```python
from build123d import *

# Parameters (mm, degrees)
SKETCH1_W               = 58
SKETCH1_H               = 38
BOSS_EXTRUDE1_DEPTH     = 1
CUT_EXTRUDE1_DEPTH      = 35.684290392
CUT_EXTRUDE1_DEPTH_BACK = 35.684290392
SKETCH2_W               = 17
SKETCH2_H               = 14.502040096
SKETCH3_W               = 3
SKETCH3_H               = 27
BOSS_EXTRUDE2_DEPTH     = 13
SKETCH4_W               = 42
SKETCH4_H               = 2
BOSS_EXTRUDE3_DEPTH     = 13
CUT_EXTRUDE2_START      = -42
SKETCH5_W               = 10
SKETCH5_H               = 5
CUT_EXTRUDE2_DEPTH      = 3
CUT_EXTRUDE3_REACH      = 39.027
SKETCH6_R               = 1.5


with BuildPart() as part:
    # Sketch1 → Boss-Extrude1 (new, symmetric)
    with BuildSketch(Plane(origin=(0, 0, 0), x_dir=(1, 0, 0), z_dir=(0, 1, 0))):
        Rectangle(SKETCH1_W, SKETCH1_H)
    extrude(amount=BOSS_EXTRUDE1_DEPTH, both=True)

    # Sketch2 → Cut-Extrude1 (cut, two sides: drawn at the far end of the back side and taken through both)
    with BuildSketch(Plane(origin=(0, 0, 0), x_dir=(1, 0, 0), z_dir=(0, 1, 0)).offset(-CUT_EXTRUDE1_DEPTH_BACK)):
        with Locations((0, 17.251020048)):
            Rectangle(SKETCH2_W, SKETCH2_H)
    extrude(amount=CUT_EXTRUDE1_DEPTH + CUT_EXTRUDE1_DEPTH_BACK, mode=Mode.SUBTRACT)

    # Sketch3 → Boss-Extrude2 (add)
    with BuildSketch(Plane(origin=(0, 1, 0), x_dir=(1, 0, 0), z_dir=(0, 1, 0))):
        with Locations((19.5, -4.5)):
            Rectangle(SKETCH3_W, SKETCH3_H)
        with Locations((-19.5, -4.5)):
            Rectangle(SKETCH3_W, SKETCH3_H)
    extrude(amount=BOSS_EXTRUDE2_DEPTH)

    # Sketch4 → Boss-Extrude3 (add)
    with BuildSketch(Plane(origin=(0, 1, 0), x_dir=(1, 0, 0), z_dir=(0, 1, 0))):
        with Locations((0, -18)):
            Rectangle(SKETCH4_W, SKETCH4_H)
    extrude(amount=BOSS_EXTRUDE3_DEPTH)

    # Sketch5 → Cut-Extrude2 (cut)
    with BuildSketch(Plane.ZY.offset(21).offset(CUT_EXTRUDE2_START)):
        with Locations((4, 5.5)):
            Rectangle(SKETCH5_W, SKETCH5_H)
    extrude(amount=CUT_EXTRUDE2_DEPTH, mode=Mode.SUBTRACT)

    # Sketch6 → Cut-Extrude3 (cut, up to next)
    with BuildSketch(Plane(origin=(0, 1, 0), x_dir=(1, 0, 0), z_dir=(0, 1, 0)), mode=Mode.PRIVATE) as cut_extrude3_sk1:
        with Locations(Location((-26, 15, 0), (0, 0, 270))):
            Circle(SKETCH6_R)
    cut_extrude3_tool1 = extrude(cut_extrude3_sk1.sketch, amount=-CUT_EXTRUDE3_REACH, mode=Mode.PRIVATE) & part.part
    # Sketch6 → Cut-Extrude3 (cut, up to next)
    with BuildSketch(Plane(origin=(0, 1, 0), x_dir=(1, 0, 0), z_dir=(0, 1, 0)), mode=Mode.PRIVATE) as cut_extrude3_sk2:
        with Locations(Location((-26, -15, 0), (0, 0, 90))):
            Circle(SKETCH6_R)
    cut_extrude3_tool2 = extrude(cut_extrude3_sk2.sketch, amount=-CUT_EXTRUDE3_REACH, mode=Mode.PRIVATE) & part.part
    # Sketch6 → Cut-Extrude3 (cut, up to next)
    with BuildSketch(Plane(origin=(0, 1, 0), x_dir=(1, 0, 0), z_dir=(0, 1, 0)), mode=Mode.PRIVATE) as cut_extrude3_sk3:
        with Locations(Location((26, -15, 0), (0, 0, 270))):
            Circle(SKETCH6_R)
    cut_extrude3_tool3 = extrude(cut_extrude3_sk3.sketch, amount=-CUT_EXTRUDE3_REACH, mode=Mode.PRIVATE) & part.part
    # Sketch6 → Cut-Extrude3 (cut, up to next)
    with BuildSketch(Plane(origin=(0, 1, 0), x_dir=(1, 0, 0), z_dir=(0, 1, 0)), mode=Mode.PRIVATE) as cut_extrude3_sk4:
        with Locations(Location((26, 15, 0), (0, 0, 90))):
            Circle(SKETCH6_R)
    cut_extrude3_tool4 = extrude(cut_extrude3_sk4.sketch, amount=-CUT_EXTRUDE3_REACH, mode=Mode.PRIVATE) & part.part
    add(cut_extrude3_tool1.solids().sort_by_distance((-26, 1, -15))[0], mode=Mode.SUBTRACT)
    add(cut_extrude3_tool2.solids().sort_by_distance((-26, 1, 15))[0], mode=Mode.SUBTRACT)
    add(cut_extrude3_tool3.solids().sort_by_distance((26, 1, 15))[0], mode=Mode.SUBTRACT)
    add(cut_extrude3_tool4.solids().sort_by_distance((26, 1, -15))[0], mode=Mode.SUBTRACT)


solid = part.part
```
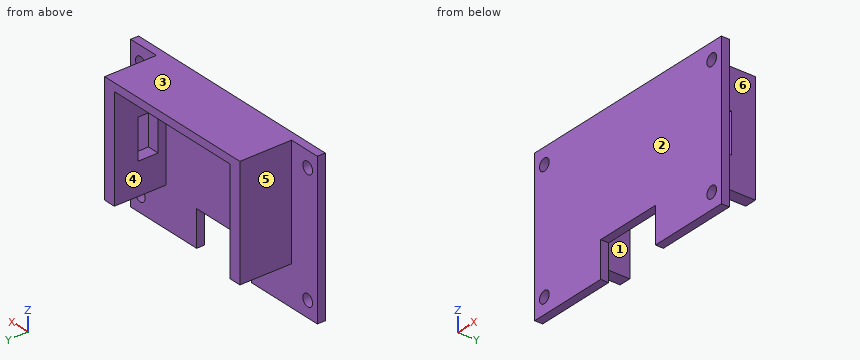
Geometry check sheet. Reference: the model listing, model coordinates, mm. Face numbers are marked on the shaded views. A direction names the side the tool comes from. Give positions to 0.01 mm unless a question says otherwise; leave off trailing zeros. Write each loop counter-clockwise with the first axis right and the second up, starting at its lowest first coordinate (ties: lowest second). Pieces come first, ordered by that corner, then holes.
1) Section check B-B, the plane y = 5.5. Record the boundary of the cut face in (x, z).
2) Access from +Z, -Z, +X, -X, +Y, -Y to the whole of each face (thin tool, end or side, straight path). Record for the marked faces 1 and 2.
3) Release check for a two-part mould opening along X. For the marked faces 3, 4, 5 and 6 record: pulls with the +X half, pulls with the -X half, needs draft (parallel to the pull), parting line crosses it, or undercut.
4) Material ranges on L1, parallel to X at y = -0.5, z = -15; L2, parallel to X at y = 10.5, z = -4.5; L3, parallel to X at y = 0, z = 15, recorded low to high.
5) Gauge pin test, flat ends, axial feed: pin 1 (2.5 mm diameter, centred on x = 26, z = -15, fed in from -Y); pin 2 (4 mm diameter, centred on y = 8, z = 2, fed in from +X); pin 3 (6.5 mm diameter, centred on x = 0, y = 5, fed in from -Z); pin 4 (2 mm diameter, centred on x = 13.5, z = -2.5, fed in from +Y). Record the tip position at first contact, or that the pin passes through.
6) Section check A-A, the plane z = 0. Record the boundary of the cut face in (x, y), and give its area (3 significant figures).
7) Section check C-C, the plane x = 26. Record the boundary of the cut face in (y, z), and give its area (3 significant figures).
8) Section check D-D, the plane z = -15. Record the boundary of the cut face in (x, y), and give its area (3 significant figures).
Computed:
1. outline: (-21, -9) - (-18, -9) - (-18, 17) - (18, 17) - (18, 9) - (21, 9) - (21, 19) - (-21, 19) - close; (18, -9) - (21, -9) - (21, -1) - (18, -1) - close
2. face 1: -Z, +Y
2. face 2: +Z, -Z, +X, -X, -Y
3. face 3: needs draft
3. face 4: undercut
3. face 5: pulls with the -X half
3. face 6: pulls with the +X half
4. L1: x = -29 to -27.5, -24.5 to -8.5, 8.5 to 24.5, 27.5 to 29
4. L2: x = -21 to -18, 18 to 21
4. L3: x = -29 to -27.5, -24.5 to 24.5, 27.5 to 29
5. pin 1: passes through
5. pin 2: stops at x = 21
5. pin 3: stops at z = 17
5. pin 4: stops at y = 1
6. outline: (-29, -1) - (29, -1) - (29, 1) - (21, 1) - (21, 3) - (18, 3) - (18, 1) - (-18, 1) - (-18, 14) - (-21, 14) - (-21, 1) - (-29, 1) - close; (18, 8) - (21, 8) - (21, 14) - (18, 14) - close
6. area: 179 mm2
7. outline: (-1, -19) - (1, -19) - (1, -16.5) - (-1, -16.5) - close; (-1, -13.5) - (1, -13.5) - (1, 13.5) - (-1, 13.5) - close; (-1, 16.5) - (1, 16.5) - (1, 19) - (-1, 19) - close
7. area: 64.0 mm2
8. outline: (-29, -1) - (-27.5, -1) - (-27.5, 1) - (-29, 1) - close; (-24.5, -1) - (-8.5, -1) - (-8.5, 1) - (-24.5, 1) - close; (8.5, -1) - (24.5, -1) - (24.5, 1) - (8.5, 1) - close; (27.5, -1) - (29, -1) - (29, 1) - (27.5, 1) - close
8. area: 70.0 mm2
